```python
from build123d import *

# Parameters (mm, degrees)
SKETCH_1_R      = 2.5
EXTRUDE_1_DEPTH = 0.5
EXTRUDE_START   = 2.75
SKETCH_2_R      = 1
EXTRUDE_2_DEPTH = 0.5
EXTRUDE_START_2 = -2.25
SKETCH_2_2_R    = 1
EXTRUDE_3_DEPTH = 0.5
FILLET_1_R      = 0.8
FILLET_2_R      = 0.5
FILLET_4_R      = 1


with BuildPart() as part:
    # Эскиз1 → Бобышка-Вытянуть1 (new body)
    with BuildSketch(Plane(origin=(0, 0, 0), x_dir=(1, 0, 0), z_dir=(0, 1, 0))):
        Polygon((-10, 4.5), (7.5, 4.5), (7.5, 1.75), (8, 1.75), (8, 2.75), (12, 2.75), (12, 1.75), (12.5, 1.75), (12.5, 4.5), (16, 4.5), (16, -4.5), (12.5, -4.5), (12.5, -1.75), (12, -1.75), (12, -2.75), (8, -2.75), (8, -1.75), (7.5, -1.75), (7.5, -4.5), (-10, -4.5), align=None)
        with Locations(Location((0, 0, 0), (0, 0, 270))):
            Circle(SKETCH_1_R, mode=Mode.SUBTRACT)
    extrude(amount=EXTRUDE_1_DEPTH)

    # Эскиз2 → Бобышка-Вытянуть2 (add)
    with BuildSketch(Plane.XY.offset(EXTRUDE_START)):
        with BuildLine():
            Line((8, 0.5), (8, 2.3))
            ThreePointArc((8, 2.3), (10, 4.3), (12, 2.3))
            Line((12, 2.3), (12, 0.5))
            Line((12, 0.5), (8, 0.5))
        make_face()
        with Locations(Location((10, 2.3, 0), (0, 0, 180))):
            Circle(SKETCH_2_R, mode=Mode.SUBTRACT)
    extrude(amount=-EXTRUDE_2_DEPTH)

    # Эскиз2<2> → Бобышка-Вытянуть3 (add)
    with BuildSketch(Plane.XY.offset(EXTRUDE_START_2)):
        with BuildLine():
            Line((8, 0.5), (8, 2.3))
            ThreePointArc((8, 2.3), (10, 4.3), (12, 2.3))
            Line((12, 2.3), (12, 0.5))
            Line((12, 0.5), (8, 0.5))
        make_face()
        with Locations(Location((10, 2.3, 0), (0, 0, 180))):
            Circle(SKETCH_2_2_R, mode=Mode.SUBTRACT)
    extrude(amount=-EXTRUDE_3_DEPTH)

    # Скругление1
    fillet_1_edges = [part.edges().sort_by_distance(p)[0] for p in [
        (-10, 0.25, 4.5),
        (-10, 0.25, -4.5),
        (16, 0.25, -4.5),
        (16, 0.25, 4.5),
    ]]
    fillet(fillet_1_edges, radius=FILLET_1_R)

    # Скругление2
    fillet_2_edges = [part.edges().sort_by_distance(p)[0] for p in [
        (10, 0.5, 2.25),
        (10, 0.5, -2.25),
    ]]
    fillet(fillet_2_edges, radius=FILLET_2_R)

    # Скругление4
    fillet_4_edges = [part.edges().sort_by_distance(p)[0] for p in [
        (10, 0, 2.75),
        (10, 0, -2.75),
    ]]
    fillet(fillet_4_edges, radius=FILLET_4_R)


solid = part.part
```
Build history of the part. All positions in model axes, mm. A direction names the side the tool comes from. Give positions to 0.01 mm unless a question says otherwise; leave off trailing zeros. Loops run counter-clockwise (first coordinate to the right, second up) from the corner with the lowest first, then second, coordinate; pieces in that order, holes last.
Item 1: Drill centre lines: line 1 (X direction, y = 2.3, z = 2.65); line 2 (Z direction, x = 9.25, y = 3.05); line 3 (Y direction, x = -8, z = 2). Where is each one in solid material? Low to high.
Answers follow:
line 1: x = 8 to 9, 11 to 12
line 2: z = -2.75 to -2.25, 2.25 to 2.75
line 3: y = 0 to 0.5
Item 2: Slice it at C-C, the plane z = 3. List the corners of the cut face in (x, y), and give its area (3 significant figures).
Answers follow:
outline: (-10, 0) - (7.5, 0) - (7.5, 0.5) - (-10, 0.5) - close; (12.5, 0) - (16, 0) - (16, 0.5) - (12.5, 0.5) - close
area: 10.5 mm2
Item 3: Which spindle directions (+Z, -Z, +X, -X, +Y, -Y) get a long thin tool onto all of the face, cutting with end or side? Do faces 1 (the face through (12, 1.2, -2.5)), 2 (the face through (9.6, 3.4, -2.25)), 3 (the face through (10.028, 0.285, -2.449)), 4 (the face through (8, 1.1, 2.5)), 5 (the face through (9.972, 0.285, 2.449)). Say none if no direction does.
Answers follow:
face 1: -Z, +Y, -Y
face 2: +X, -X, +Y
face 3: -Z, -Y
face 4: +Z, +Y, -Y
face 5: +Z, -Y
Item 4: Slice it at B-B, the plane x = 0. List the corners of the cut face in (y, z), and give its area (3 significant figures).
Answers follow:
outline: (0, -4.5) - (0.5, -4.5) - (0.5, -2.5) - (0, -2.5) - close; (0, 2.5) - (0.5, 2.5) - (0.5, 4.5) - (0, 4.5) - close
area: 2.00 mm2
Item 5: Slice it at A-A, the plane y = 1.7. List the corners of the cut face in (x, z).
Answers follow:
outline: (8, -2.75) - (9.2, -2.75) - (9.2, -2.25) - (8, -2.25) - close; (8, 2.25) - (9.2, 2.25) - (9.2, 2.75) - (8, 2.75) - close; (10.8, -2.75) - (12, -2.75) - (12, -2.25) - (10.8, -2.25) - close; (10.8, 2.25) - (12, 2.25) - (12, 2.75) - (10.8, 2.75) - close
Item 6: Flat gauge pins, fed straight in: pin 1 (1.8 mm diameter, centred on x = 10, y = 2.3, fed in from +Z); pin 2 (0.6 mm diameter, centred on x = 8, y = 0, fed in from +Z); pin 3 (2.5 mm diameter, centred on x = 9, y = 2.5, fed in from +Z); pin 4 (3 mm diameter, centred on x = -1, z = 1, fed in from -Y). Where does each tip first touch, or does it go through?
Answers follow:
pin 1: passes through
pin 2: stops at z = 2.46
pin 3: stops at z = 2.75
pin 4: stops at y = 0
Item 7: Slice it at D-D, the plane x = 10. List the corners of the cut face in (y, z), and give its area (3 significant figures).
Answers follow:
outline: (0, -1.75) arc R1 ccw to (1, -2.75) - (1.3, -2.75) - (1.3, -2.25) - (1, -2.25) arc R0.5 cw to (0.5, -1.75) - (0.5, 1.75) arc R0.5 cw to (1, 2.25) - (1.3, 2.25) - (1.3, 2.75) - (1, 2.75) arc R1 ccw to (0, 1.75) - close; (3.3, -2.75) - (4.3, -2.75) - (4.3, -2.25) - (3.3, -2.25) - close; (3.3, 2.25) - (4.3, 2.25) - (4.3, 2.75) - (3.3, 2.75) - close
area: 4.23 mm2
Item 8: Pull direction Z, two halves, no side cores. Call faces 6 (the face through (11, 2.3, -2.5)), 7 (the face through (9.6, 3.4, -2.75)), 8 (the face through (-2.44, 0.25, -0.54)): released by +Z, released by -Z, zero draft, split by the parting line, or undercut.
Answers follow:
face 6: zero draft
face 7: released by -Z
face 8: undercut
